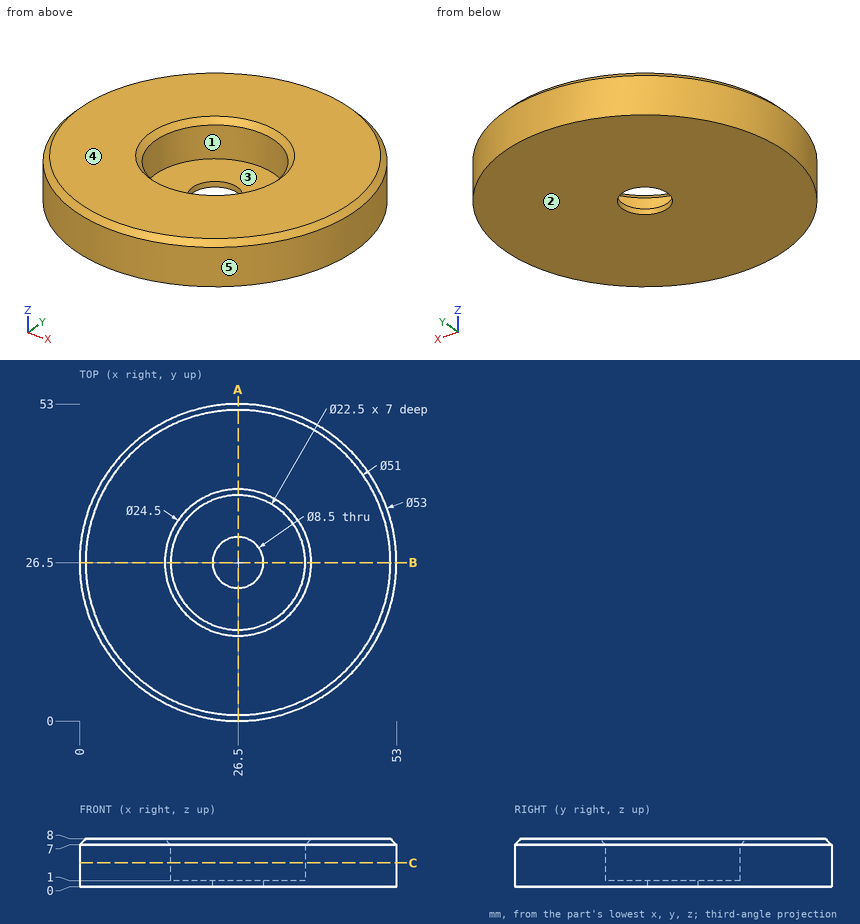
Answer from the drawing. Dimensions are ordinates in mm from the lowest x, y and z of the part. A direction names the side the tool comes from. Give positions to 0.01 mm unless a question says otherwise; leave off trailing zeros. Order: outer loops, then holes, each group sorted by start corner. A loop starts at its lowest first (then second) coordinate and runs counter-clockwise, first axis right, second up. Notation, with made-up numbers: (-30.75, 18.5) - (8.25, 18.5) arc R18 ccw to (8.25, 28.5) - close; hole circle Ø4 at (61, 50.25). An arc over 180 degrees is marked (long way). Use one line per item in the form item = value.
1) Each of these flat-tipped pins is pushed along its axis until it touches: pin 1 (11 mm diameter, centred on x = 26.5, y = 26.5, fed in from +Z); pin 2 (1.5 mm diameter, centred on x = 17, z = 1, fed in from -Y); pin 3 (4 mm diameter, centred on x = 30, z = 2.5, fed in from +Y). Where does it stop, or does it pass through?
Verdict:
pin_1 = 1
pin_2 = 1.49
pin_3 = 52.96
2) Find section A-A on x = 26.5. Determine the outline of the cut face in (y, z).
Verdict:
outline = (0, 0) - (22.25, 0) - (22.25, 1) - (15.25, 1) - (15.25, 7) - (14.25, 8) - (1, 8) - (0, 7) - close; (30.75, 0) - (53, 0) - (53, 7) - (52, 8) - (38.75, 8) - (37.75, 7) - (37.75, 1) - (30.75, 1) - close
3) The mould has two halves that part along Y. Classify the marked faces 3, 4 and 5: released by +Y, released by -Y, zero draft, split by the parting line, or undercut.
Verdict:
face_3 = undercut
face_4 = zero draft
face_5 = split by the parting line
4) For the marked faces 1 and 2, determine the directions among +Z, -Z, +X, -X, +Y, -Y from which every point of the face is accessible in a straight line to the end or side of a thin tool.
Verdict:
face_1 = +Z
face_2 = -Z, +X, -X, +Y, -Y
5) Consider probe 1 along Y at (x, z) = (26.5, 4.05); probe 2 along Z at (x, y) = (36, 22.5); probe 3 along Y at (x, z) = (26.5, 0.35). Determine where each line is inside the solid, lowest interval first. Write a range as [from, to].
Verdict:
probe_1 = [0, 15.25], [37.75, 53]
probe_2 = [0, 1]
probe_3 = [0, 22.25], [30.75, 53]
6) Find section C-C on z = 4. Determine the outline of the cut face in (x, y), and give its area (3 significant figures).
Verdict:
outline = circle Ø53 at (26.5, 26.5); hole circle Ø22.5 at (26.5, 26.5)
area = 1,810 mm^2
